Autodesk Inventor part; units mm, degrees
ref_plane "CP_XY" through (0, 0, 0) normal (1, 0, 0) x (0, 0, -1)
ref_plane "CP_YZ" through (0, 0, 0) normal (0, 0, -1) x (0, 1, 0)
ref_plane "CP_ZX" through (0, 0, 0) normal (0, 1, 0) x (1, 0, 0)
sketch "Sketch_1" plane through (0, 0, 0) normal (0, 0, 1) x (1, 0, 0)
  line L0 (0, 0) -> (-10, 0)
  line L1 (-10, 0) -> (-10, 3.233)
  line L2 (-10, 3.233) -> (-9.233, 4)
  line L3 (-9.233, 4) -> (-1.25, 4)
  line L4 (-1.25, 4) -> (0, 2.75)
  line L5 (0, 2.75) -> (0, 0)
  line L6 (0, 0) -> (-10, 0)
revolve "Revolution1" add sketch "Sketch_1" angle 360 about axis through (0, 0, 0) along (1, 0, 0)
thread "Thread1"
sketch "Sketch_2" plane through (-10, 0, 0) normal (-1, 0, 0) x (0, 1, 0)
  line L0 (-2, -1.1547) -> (0, -2.3094)
  line L1 (0, -2.3094) -> (2, -1.1547)
  line L2 (2, -1.1547) -> (2, 1.1547)
  line L3 (2, 1.1547) -> (0, 2.3094)
  line L4 (0, 2.3094) -> (-2, 1.1547)
  line L5 (-2, 1.1547) -> (-2, -1.1547)
extrude "Extrusion1" cut sketch "Sketch_2" against normal blind 3
sketch "Sketch_3" plane through (0, 0, 0) normal (0, 0, 1) x (1, 0, 0)
  line L0 (-5.8453, 0) -> (-7, 0)
  line L1 (-7, 0) -> (-7, 2)
  line L2 (-7, 2) -> (-5.8453, 0)
  line L3 (-5.8453, 0) -> (-7, 0)
revolve "Revolution2" cut sketch "Sketch_3" angle 360 about axis through (-5.8453, 0, 0) along (1, 0, 0)
ref_plane "CP_XY" through (0, 0, 0) normal (1, 0, 0) x (0, 0, -1)
ref_plane "CP_YZ" through (0, 0, 0) normal (0, 0, -1) x (0, 1, 0)
ref_plane "CP_ZX" through (0, 0, 0) normal (0, 1, 0) x (1, 0, 0)
properties part number "SET-SCREW8-10"
Part model, mm, in its own coordinate system. A direction names the side the tool comes from. Round coordinates to 2 decimals unless told otherwise and drop trailing zeros. Loops run counter-clockwise (first coordinate to the right, second up) from the corner with the lowest first, then second, coordinate; pieces in that order, holes last. Notation, with made-up numbers: (49.25, 3.5) -> (105.25, 3.5) arc R16 cw to (105.25, 8.5) -> close; hole circle Ø1 at (7.5, -1.75). An arc over 180 degrees is marked (long way). Use a Markdown table: item, result.
1) Drop flat-ended pins along their axis: pin 1 Ø1.5 at (x, z) = (-2, 1.5) entering from -Y; pin 2 Ø3 at (x, z) = (-3, -2) entering from +Y; pin 3 Ø2 at (x, z) = (-3, 3) entering from -Y. Give the stop position or say it passes through.
The answers:
| item | result |
|---|---|
| pin 1 | stops at y = -3.93 |
| pin 2 | stops at y = 3.97 |
| pin 3 | stops at y = -3.46 |
2) Probe line 1 (Z direction, x = -9.5, y = 1); line 2 (Y direction, x = -6.75, z = 0.25); line 3 (Z direction, x = -8.75, y = 0.5). List the from-to ranges inside material, lowest first. Write a range as [from, to].
The answers:
| item | result |
|---|---|
| line 1 | z = [-3.6, -1.73], [1.73, 3.6] |
| line 2 | y = [-3.99, -1.55], [1.55, 3.99] |
| line 3 | z = [-3.97, -2.02], [2.02, 3.97] |
3) Tool access for faces 4 (the flat face through (-8.521, 1.014, -1.724)), 5 (the flat face through (0, 0, 0)): list every direction of +Z, -Z, +X, -X, +Y, -Y with a clear straight run to the whole face (end or side of a thin tool).
The answers:
| item | result |
|---|---|
| face 4 | -X |
| face 5 | +Z, -Z, +X, +Y, -Y |
4) Cut at A-A, the plane x = -1. List the corners of the cut face in (y, z).
The answers:
| item | result |
|---|---|
| outline | circle Ø7.5 at (0, 0) |
5) Pull direction Z, two halves, no side cores. Call faces 1 (the flat face through (-10, 1, -2)), 2 (the cylindrical face through (-5.186, -0.867, -3.905)), 3 (the flat face through (-8.52, 0.99, 1.74)): pulls with the +Z half, pulls with the -Z half, needs draft (parallel to the pull), parting line crosses it, or undercut.
The answers:
| item | result |
|---|---|
| face 1 | needs draft |
| face 2 | parting line crosses it |
| face 3 | undercut |
